Autodesk Inventor part; units mm, degrees
ref_plane "YZ Plane" through (0, 0, 0) normal (1, 0, 0) x (0, 1, 0)
ref_plane "XZ Plane" through (0, 0, 0) normal (0, 1, 0) x (-1, 0, 0)
ref_plane "XY Plane" through (0, 0, 0) normal (0, 0, 1) x (1, 0, 0)
sketch "Sketch1" plane through (0, 0, 0) normal (0, 0, 1) x (1, 0, 0)
  circle A0 centre (0, 0) radius 1.5
  circle A1 centre (0, 0) radius 5
  line L0 (0, 5) -> (-17.5, 5)
  circle A2 centre (-17.5, 0) radius 5
  line L1 (-17.5, -5) -> (0, -5)
  line L2 (-17.5, 0) -> (0, 0)
  line L3 (-17.5, 5) -> (-22.5, 5)
  line L4 (-22.5, 5) -> (-22.5, -5)
  line L5 (-22.5, -5) -> (-17.5, -5)
  line L6 (-1.118, 1) -> (1.118, 1)
  line L7 (0, 1) -> (0, -1.5)
  point P0 (-22.5, 0)
  dimension "d0" = 3
  dimension "d1" = 3.5
  dimension "d3" = 17.5
  dimension "d12" = 2.5
extrude "Extrusion1" add sketch "Sketch1" along normal blind 4 contours A1 | A1 L1 A2 L2 | L2 A2 L0 A1 | L6 A0 | A2 | A2 L4 L3 | L5 L4 A2
fillet "Fillet1" radius 1.5 2 edges at (-22.5, 5, 2) (-22.5, -5, 2)
sketch "Sketch3" plane through (0, 0, 0) normal (0, 0, -1) x (-1, 0, 0)
  arc A0 (21, -5) -> (22.5, -3.5) centre (21, -3.5) ccw
  line L0 (21, -5) -> (0, -5)
  arc A1 (0, 5) -> (0, -5) centre (0, 0) ccw
  line L1 (0, 5) -> (21, 5)
  arc A2 (22.5, 3.5) -> (21, 5) centre (21, 3.5) ccw
  line L2 (22.5, 3.5) -> (22.5, -3.5)
  arc A3 (-1.118, 1) -> (1.118, 1) centre (0, 0) ccw
  line L3 (0, 5) -> (21, 5)
  arc A4 (22.5, 3.5) -> (21, 5) centre (21, 3.5) ccw
  line L4 (15.5, 5) -> (15.5, -5)
  line L5 (21, -5) -> (0, -5)
  line L6 (1.118, 1) -> (-1.118, 1)
  dimension "d8" = 7
extrude "Extrusion2" add sketch "Sketch3" along normal blind 16 contours L0 L4 L1 A2 L2 A0
fillet "Fillet2" radius 2 1 edges at (-15.5, 0, 0)
properties part number "AcoplePPR"
Read the model definition and answer for the solid it produces. Units are mm, in the model's axes. A direction names the side the tool comes from. Give positions to 0.01 mm unless a question says otherwise; leave off trailing zeros. Loops run counter-clockwise (first coordinate to the right, second up) from the corner with the lowest first, then second, coordinate; pieces in that order, holes last. Notation, with made-up numbers: (59, -13) -> (116, -13) arc R20 ccw to (116, -9) -> close; hole circle Ø6 at (41.5, 2.25). An arc over 180 degrees is marked (long way). Answer as CSV lines item,"result".
Item 1: Find section D-D on x = -9.5. Give the vertices of the cut face in (y, z), plus the area to 3 significant figures.
Returned:
outline,"(-5, 0) -> (5, 0) -> (5, 4) -> (-5, 4) -> close"
area,"40.0 mm²"
Item 2: Find section B-B on z = -8.5. Give the vertices of the cut face in (x, y).
Returned:
outline,"(-22.5, -3.5) arc R1.5 ccw to (-21, -5) -> (-15.5, -5) -> (-15.5, 5) -> (-21, 5) arc R1.5 ccw to (-22.5, 3.5) -> close"
Item 3: Consider line 1 (Y direction, x = 0, z = 0.9); line 2 (X direction, y = 0, z = 0.8); line 3 (Z direction, x = -7, y = 4). Determine where each line is inside the solid, lowest interval first. Write a range as [from, to].
Returned:
line 1,"y = [-5, -1.5], [1, 5]"
line 2,"x = [-22.5, -1.5], [1.5, 5]"
line 3,"z = [0, 4]"
Item 4: Determine the mould class of faces 1 (the face through (5, 0, 2)), 2 (the face through (0, 1, 2)), 3 (the face through (0, -1.5, 2)), 4 (the face through (-4, 0, 0)) for opening direction Y: +Y half, -Y half, draft (parallel to the pull), parting line (faces both ways), or undercut.
Returned:
face 1,"parting line"
face 2,"undercut"
face 3,"undercut"
face 4,"draft"
Item 5: Find section C-C on y = -2.75. Give the vertices of the cut face in (x, z), plus the area to 3 significant figures.
Returned:
outline,"(-22.5, -16) -> (-15.5, -16) -> (-15.5, -2) arc R2 cw to (-13.5, 0) -> (4.18, 0) -> (4.18, 4) -> (-22.5, 4) -> close"
area,"220 mm²"
Item 6: For faces 5 (the face through (-15.5, 0, -9)), 6 (the face through (-22.05, 4.57, -5.86)), determine the directions among +Z, -Z, +X, -X, +Y, -Y from which every point of the face is accessible in a straight line to the end or side of a thin tool.
Returned:
face 5,"-Z, +X, +Y, -Y"
face 6,"+Z, -Z, -X, +Y"
Item 7: Each of these flat-tipped pins is pushed along its axis until it touches: pin 1 (1 mm diameter, centred on y = 2, z = -12.5, fed in from +X); pin 2 (2 mm diameter, centred on x = -13.5, y = -2, fed in from -Z); pin 3 (2.5 mm diameter, centred on x = 0, y = 0, fed in from -Z). Where does it stop, or does it pass through?
Returned:
pin 1,"stops at x = -15.5"
pin 2,"stops at z = -0.27"
pin 3,"stops at z = 0"
Item 8: Find section A-A on y = 0. Give the vertices of the cut face in (x, z).
Returned:
outline,"(-22.5, -16) -> (-15.5, -16) -> (-15.5, -2) arc R2 cw to (-13.5, 0) -> (-1.5, 0) -> (-1.5, 4) -> (-22.5, 4) -> close; (1.5, 0) -> (5, 0) -> (5, 4) -> (1.5, 4) -> close"
